from build123d import *

# Parameters (mm, degrees)
F2_R            = 7
F3_DEPTH        = 25
F3_COPIES_COUNT = 6


# Not quite as in the source:
# - a pattern or mirror of a feature is missing from the dataset's text; its kind, count and spacing are read off the source's solid


with BuildPart() as f1:
    # F0 (on Right) → F1 (revolve)
    with BuildSketch(Plane.YZ):
        with BuildLine():
            Line((160, 16), (125, 16))
            Line((125, 16), (115.9647238196, 13.5790050441))
            ThreePointArc((115.9647238196, 13.5790050441), (113.8265866388, 12.1503474549), (113, 9.7153017389))
            Line((113, 9.7153017389), (113, 0))
            Line((113, 0), (160, 0))
            Line((160, 0), (160, 16))
        make_face()
    revolve(axis=Axis((0, 0, -1.8696532477), (0, 0, -1)))

    # F2 (on face) → F3 (cut)
    with BuildSketch(Plane.XY.offset(16)):
        with Locations((0, 140)):
            Circle(F2_R)
    f3 = extrude(amount=-F3_DEPTH, mode=Mode.SUBTRACT)

    # F3_copies: F3 ×6 about axis
    f3_copies_axis = Axis((0, 0, 0), (0, 0, 1))
    for i in range(1, F3_COPIES_COUNT):
        add(f3.rotate(f3_copies_axis, i * 360 / F3_COPIES_COUNT), mode=Mode.SUBTRACT)


solid = f1.part
Model file for the job. Use its own axes, mm. Coordinates: 2 decimals unless noted, no trailing zeros. Order: outer loops, then holes, each group sorted by start corner. A loop starts at its lowest first (then second) coordinate and runs counter-clockwise, first axis right, second up. Notation, with made-up numbers: (43, 8.25) -> (76, 8.25) arc R17 ccw to (76, 36.25) -> close; hole circle Ø2 at (2.25, 79.25). An arc over 180 degrees is marked (long way). Return JSON: item names as keys, results as strings. Group by question number.
Item 1: Saw through at B-B on y = 0. Write the cut outline in (x, z).
Item 2: Pull direction X, two halves, no side cores. Call faces 1 (the cylindrical face through (-156.195, -34.685, 8.112)), 2 (the conical face through (-113.635, -25.234, 13.697)), 3 (the flat face through (96, 82, 16)): pulls with the +X half, pulls with the -X half, needs draft (parallel to the pull), parting line crosses it, or undercut.
Item 3: Wall check: line 1 along Y through (x, z) = (4.5, 12); line 2 along Y through (x, z) = (120.5, 11); line 3 along X through (y, z) = (-69.5, 2.5). Give the ranges that are in metal, low to high. Write a range as [from, to].
Item 4: Flat gauge pins, fed straight in: P1, Ø3, axis at y = 14, z = 12.5, coming from the -X side; P2, Ø4, axis at y = 44, z = 2, coming from the +X side; P3, Ø2, axis at y = 26, z = 9, coming from the +X side. Where does each tip first touch, or does it go through?
Item 5: Saw through at A-A on x = 0. Write the cut outline in (y, z), then the cut area to 3 significant figures.
Item 6: Saw through at D-D on y = 70. State how many separate pieces and enclosed holes the cut face has, then the cut area to 3 significant figures.
Item 7: Saw through at C-C on z = 5.25. Write the cut outline in (x, y).
Values found:
{
 "1": {"outline": "(-160, 0) -> (-113, 0) -> (-113, 9.72) arc R4 ccw to (-115.96, 13.58) -> (-125, 16) -> (-160, 16) -> close; (113, 0) -> (160, 0) -> (160, 16) -> (125, 16) -> (115.96, 13.58) arc R4 ccw to (113, 9.72) -> close"},
 "2": {"face 1": "parting line crosses it", "face 2": "undercut", "face 3": "needs draft"},
 "3": {"line 1": "y = [-159.94, -145.36], [-134.64, -113.63], [113.63, 134.64], [145.36, 159.94]", "line 2": "y = [-105.26, -76.96], [-63.04, 63.04], [76.96, 105.26]", "line 3": "x = [-144.12, -128.23], [-114.26, -89.1], [89.1, 114.26], [128.23, 144.12]"},
 "4": {"P1": "stops at x = -159.51", "P2": "stops at x = 154.39", "P3": "stops at x = 158.03"},
 "5": {"outline": "(-160, 0) -> (-147, 0) -> (-147, 16) -> (-160, 16) -> close; (-133, 0) -> (-113, 0) -> (-113, 9.72) arc R4 ccw to (-115.96, 13.58) -> (-125, 16) -> (-133, 16) -> close; (113, 0) -> (133, 0) -> (133, 16) -> (125, 16) -> (115.96, 13.58) arc R4 ccw to (113, 9.72) -> close; (147, 0) -> (160, 0) -> (160, 16) -> (147, 16) -> close", "area": "1,010 mm2"},
 "6": {"separate pieces": "4", "enclosed holes": "0", "area": "1,260 mm2"},
 "7": {"outline": "circle Ø320 at (0, 0); hole circle Ø14 at (-121.24, -70); hole circle Ø14 at (-121.24, 70); hole circle Ø226 at (0, 0); hole circle Ø14 at (0, -140); hole circle Ø14 at (0, 140); hole circle Ø14 at (121.24, -70); hole circle Ø14 at (121.24, 70)"}
}
